from build123d import *

# Parameters (mm, degrees)
SCHIZZO1_W                   = 20
SCHIZZO1_H                   = 100
ESTRUSIONE_ESTRUSIONE1_DEPTH = 1
SCHIZZO2_W                   = 1
SCHIZZO2_H                   = 100
ESTRUSIONE_ESTRUSIONE2_DEPTH = 90
SCHIZZO3_R                   = 2.5
TAGLIO_ESTRUSIONE1_DEPTH     = 42
SCHIZZO4_R                   = 2.5
TAGLIO_ESTRUSIONE2_DEPTH     = 42


with BuildPart() as part:
    # Schizzo1 → Estrusione-Estrusione1 (new body)
    with BuildSketch(Plane(origin=(0, 0, 0), x_dir=(1, 0, 0), z_dir=(0, 1, 0))):
        with Locations((10, -50)):
            Rectangle(SCHIZZO1_W, SCHIZZO1_H)
    extrude(amount=ESTRUSIONE_ESTRUSIONE1_DEPTH)

    # Schizzo2 → Estrusione-Estrusione2 (add)
    with BuildSketch(Plane(origin=(0, 1, 0), x_dir=(1, 0, 0), z_dir=(0, 1, 0))):
        with Locations((0.5, -50)):
            Rectangle(SCHIZZO2_W, SCHIZZO2_H)
    extrude(amount=ESTRUSIONE_ESTRUSIONE2_DEPTH)

    # Schizzo3 → Taglio-Estrusione1 (cut)
    with BuildSketch(Plane(origin=(0, 1, 0), x_dir=(1, 0, 0), z_dir=(0, 1, 0))):
        with Locations((10, -90)):
            Circle(SCHIZZO3_R)
        with Locations((10, -50)):
            Circle(SCHIZZO3_R)
        with Locations((10, -10)):
            Circle(SCHIZZO3_R)
    extrude(amount=-TAGLIO_ESTRUSIONE1_DEPTH, mode=Mode.SUBTRACT)

    # Schizzo4 → Taglio-Estrusione2 (cut)
    with BuildSketch(Plane(origin=(1, 0, 0), x_dir=(0, 0, -1), z_dir=(1, 0, 0))):
        with Locations((-30, 70)):
            Circle(SCHIZZO4_R)
        with Locations((-80, 70)):
            Circle(SCHIZZO4_R)
    extrude(amount=-TAGLIO_ESTRUSIONE2_DEPTH, mode=Mode.SUBTRACT)


solid = part.part
Work out the finished part from the listing and answer in its coordinate system (mm). A direction names the side the tool comes from. Give positions to 0.01 mm unless a question says otherwise; leave off trailing zeros. Loops run counter-clockwise (first coordinate to the right, second up) from the corner with the lowest first, then second, coordinate; pieces in that order, holes last. Notation, with made-up numbers: (-21, 27) - (29, 27) arc R24 cw to (29, 61) - close; hole circle Ø7 at (7.5, -27). An arc over 180 degrees is marked (long way). Answer in a Markdown table with one row per item.
(1) Section C-C (z = 80) is taken. Give the vertices of the cut face in (x, y).
Results list:
| item | result |
|---|---|
| outline | (0, 0) - (20, 0) - (20, 1) - (1, 1) - (1, 67.5) - (0, 67.5) - close; (0, 72.5) - (1, 72.5) - (1, 91) - (0, 91) - close |
(2) Flat-ended cylindrical pins translate along their axes: pin 1 Ø6 at (x, y) = (5.5, 27) entering from +Z; pin 2 Ø3 at (x, z) = (14.5, 17) entering from +Y. Find the tip coordinate at first contact, or state that the pin passes through.
Results list:
| item | result |
|---|---|
| pin 1 | passes through |
| pin 2 | stops at y = 1 |
(3) Section B-B (y = 70) is taken. Give the vertices of the cut face in (x, z).
Results list:
| item | result |
|---|---|
| outline | (0, 0) - (1, 0) - (1, 27.5) - (0, 27.5) - close; (0, 32.5) - (1, 32.5) - (1, 77.5) - (0, 77.5) - close; (0, 82.5) - (1, 82.5) - (1, 100) - (0, 100) - close |
(4) Section A-A (x = 10) is taken. Give the vertices of the cut face in (y, z), and give its area (3 significant figures).
Results list:
| item | result |
|---|---|
| outline | (0, 0) - (1, 0) - (1, 7.5) - (0, 7.5) - close; (0, 12.5) - (1, 12.5) - (1, 47.5) - (0, 47.5) - close; (0, 52.5) - (1, 52.5) - (1, 87.5) - (0, 87.5) - close; (0, 92.5) - (1, 92.5) - (1, 100) - (0, 100) - close |
| area | 85.0 mm² |
(5) Section D-D (z = 17) is taken. Give the vertices of the cut face in (x, y).
Results list:
| item | result |
|---|---|
| outline | (0, 0) - (20, 0) - (20, 1) - (1, 1) - (1, 91) - (0, 91) - close |
(6) A tool of negligible diameter and unlimited length cuts with its end or side. For faces 5 (the face through (1, 45, 51)), 6 (the face through (9.67, 0.51, 87.52)), from which of +Z, -Z, +X, -X, +Y, -Y can it reach the whole face along a straight path? Write none if from no direction.
Results list:
| item | result |
|---|---|
| face 5 | +Z, -Z, +X, +Y |
| face 6 | +Y, -Y |
(7) Consider L1, parallel to Y at x = 0.8, z = 80; L2, parallel to Y at x = 13.25, z = 39; L3, parallel to X at y = 0.6, z = 10. Determine where each line is inside the solid, lowest interval first. Write a range as [from, to].
Results list:
| item | result |
|---|---|
| L1 | y = [0, 67.5], [72.5, 91] |
| L2 | y = [0, 1] |
| L3 | x = [0, 7.5], [12.5, 20] |
(8) For a pull along Z with two mould halves and no side action, classify faces 1 (the face through (15, 1, 49)), 2 (the face through (0.51, 67.56, 30.54)), 3 (the face through (0.3, 45.3, 0)), 4 (the face through (0.5, 68.5, 82)) as pulls with the +Z half, pulls with the -Z half, needs draft (parallel to the pull), parting line crosses it, or undercut.
Results list:
| item | result |
|---|---|
| face 1 | needs draft |
| face 2 | undercut |
| face 3 | pulls with the -Z half |
| face 4 | undercut |
